Answer from the drawing. Dimensions are ordinates in mm from the lowest x, y and z of the part. A direction names the side the tool comes from. Coordinates: 2 decimals unless noted, no trailing zeros. Write each loop counter-clockwise with the first axis right and the second up, starting at its lowest first coordinate (ties: lowest second). Pieces come first, ordered by that corner, then holes.
1) Which of the six approach directions +Z, -Z, +X, -X, +Y, -Y give full straight-line access (tool end or side, diameter ignored) to the marked faces 1, 2 and 3?
2) Find the intervals of material crossed by line 1 (X direction, y = 28.5, z = 11.5); line 2 (Z direction, x = 5.5, y = 23.5); line 3 (Y direction, x = 12, z = 14), in increasing order.
3) Each of these flat-tipped pins is pushed along its axis until it touches: pin 1 Ø12 at (y, z) = (4.5, 12.5) entering from -X; pin 2 Ø3.5 at (x, y) = (5.47, 20) entering from +Z; pin 3 Ø5 at (x, z) = (12, 28) entering from -Y; pin 4 Ø16 at (y, z) = (17, 22) entering from +X. Where does it stop, or does it pass through?
4) The part is cut by section B-B (y = 27). Determine the outline of the cut face in (x, z) (1 decimal).
5) The part is cut by section D-D (z = 7). Determine the outline of the cut face in (x, y).
6) The part is cut by section A-A (x = 20). Determine the outline of the cut face in (y, z), then the cut area to 3 significant figures.
7) The part is cut by section C-C (x = 4.5). Determine the outline of the cut face in (y, z).
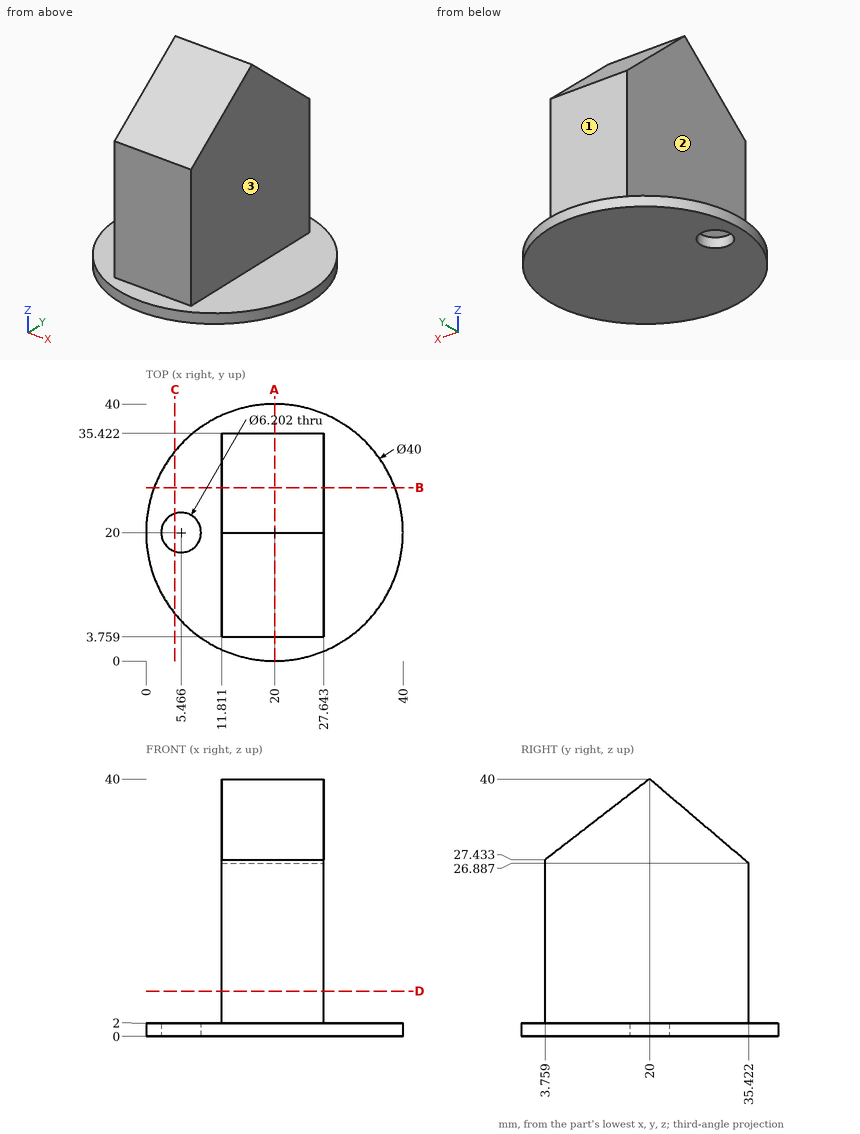
Reported:
1. face 1: +Z, +X, -X, +Y
1. face 2: +Z, -X, +Y, -Y
1. face 3: +Z, +X, +Y, -Y
2. line 1: x = 11.81 to 27.64
2. line 2: z = 0 to 2
2. line 3: y = 3.76 to 35.42
3. pin 1: stops at x = 11.81
3. pin 2: passes through
3. pin 3: stops at y = 3.76
3. pin 4: stops at x = 27.64
4. outline: (1.3, 0) - (38.7, 0) - (38.7, 2) - (27.6, 2) - (27.6, 34) - (11.8, 34) - (11.8, 2) - (1.3, 2) - close
5. outline: (11.81, 3.76) - (27.64, 3.76) - (27.64, 35.42) - (11.81, 35.42) - close
6. outline: (0, 0) - (40, 0) - (40, 2) - (35.42, 2) - (35.42, 26.89) - (20, 40) - (3.76, 27.43) - (3.76, 2) - (0, 2) - close
6. area: 1,080 mm2
7. outline: (7.36, 0) - (17.05, 0) - (17.05, 2) - (7.36, 2) - close; (22.95, 0) - (32.64, 0) - (32.64, 2) - (22.95, 2) - close
